```python
from build123d import *

# Parameters (mm, degrees)
EXTRUDE_2_DEPTH     = 9.8
CUT_EXTRUDE_1_DEPTH = 3
CUT_EXTRUDE_2_DEPTH = 2.5


with BuildPart() as part:
    # 草图1 → 凸台-拉伸2 (new body)
    with BuildSketch(Plane(origin=(0, 0, 0), x_dir=(1, 0, 0), z_dir=(0, 1, 0))):
        with BuildLine():
            Line((4.583240997, 11.690443213), (4.583240997, 14.234072022))
            Line((4.583240997, 14.234072022), (1.518891733, 14.234072022))
            ThreePointArc((1.518891733, 14.234072022), (-1.351843031, 11.65188196), (-2.416759003, 7.940443213))
            Line((-2.416759003, 7.940443213), (-2.416759003, 5.734072022))
            Line((-2.416759003, 5.734072022), (-5.066759003, 5.734072022))
            Line((-5.066759003, 5.734072022), (-5.066759003, -14.065927978))
            Line((-5.066759003, -14.065927978), (-3.166759003, -14.065927978))
            Line((-3.166759003, -14.065927978), (-3.166759003, -7.864819945))
            ThreePointArc((-3.166759003, -7.864819945), (-0.896836557, -2.38474239), (4.583240997, -0.114819945))
            Line((4.583240997, -0.114819945), (4.583240997, 4.190443213))
            ThreePointArc((4.583240997, 4.190443213), (0.833240997, 7.940443213), (4.583240997, 11.690443213))
        make_face()
        with BuildLine():
            ThreePointArc((11.583240997, 7.940443213), (10.518325026, 11.65188196), (7.647590262, 14.234072022))
            Line((7.647590262, 14.234072022), (4.583240997, 14.234072022))
            Line((4.583240997, 14.234072022), (4.583240997, 11.690443213))
            ThreePointArc((4.583240997, 11.690443213), (7.234891427, 10.592093643), (8.333240997, 7.940443213))
            ThreePointArc((8.333240997, 7.940443213), (7.234891427, 5.288792784), (4.583240997, 4.190443213))
            Line((4.583240997, 4.190443213), (4.583240997, -0.114819945))
            ThreePointArc((4.583240997, -0.114819945), (10.063318551, -2.38474239), (12.333240997, -7.864819945))
            Line((12.333240997, -7.864819945), (12.333240997, -14.065927978))
            Line((12.333240997, -14.065927978), (14.233240997, -14.065927978))
            Line((14.233240997, -14.065927978), (14.233240997, 5.734072022))
            Line((14.233240997, 5.734072022), (11.583240997, 5.734072022))
            Line((11.583240997, 5.734072022), (11.583240997, 7.940443213))
        make_face()
    extrude(amount=EXTRUDE_2_DEPTH)

    # 草图2 → 切除-拉伸1 (cut)
    with BuildSketch(Plane(origin=(0, 9.8, 0), x_dir=(1, 0, 0), z_dir=(0, 1, 0))):
        Polygon((-7.578838201, -4.016286107), (16.085093039, -4.259527691), (16.085093039, 14.991306239), (-7.578838201, 14.991306239), align=None)
    extrude(amount=-CUT_EXTRUDE_1_DEPTH, mode=Mode.SUBTRACT)

    # 草图3 → 切除-拉伸2 (cut)
    with BuildSketch(Plane(origin=(0, 6.8, 0), x_dir=(1, 0, 0), z_dir=(0, 1, 0))):
        Polygon((-9.750638057, 0), (19.90166932, 0), (19.90166932, 15.470839647), (-9.750638057, 15.762729548), align=None)
    extrude(amount=-CUT_EXTRUDE_2_DEPTH, mode=Mode.SUBTRACT)


solid = part.part
```
Work out the finished part from the listing and answer in its coordinate system (mm). A direction names the side the tool comes from. Round coordinates to 2 decimals unless told otherwise and drop trailing zeros. Write each loop counter-clockwise with the first axis right and the second up, starting at its lowest first coordinate (ties: lowest second). Pieces come first, ordered by that corner, then holes. Notation, with made-up numbers: (-5.75, -37) - (22.25, -37) arc R30 ccw to (22.25, -2) - close; hole circle Ø5 at (41.25, -36.75). An arc over 180 degrees is marked (long way). Return JSON: item names as keys, results as strings. Group by question number.
Q1. The part is cut by section D-D on x = 5.75. Write down the section's boundary in (y, z), then the cut area to 3 significant figures.
Q2. The part is cut by section C-C on y = 8.25. Write down the section's boundary in (x, z).
Q3. The part is cut by section A-A on y = 1.5. Write down the section's boundary in (x, z), then the cut area to 3 significant figures.
Q4. The part is cut by section B-B on z = 9.75. Write down the section's boundary in (x, y).
Q5. For faces 1 (the flat face through (13, 2, -5.734)), 2 (the flat face through (-4, 5, 14.066)), 3 (the flat face through (4, 4.3, -4)), 4 (the flat face through (-3.167, 5, 11)), 5 (the flat face through (-2.417, 2, -7)), determine the directions among +Z, -Z, +X, -X, +Y, -Y from which every point of the face is accessible in a straight line to the end or side of a thin tool.
Q6. Each of these flat-tipped pins is pushed along its axis until it touches: pin 1 Ø4 at (y, z) = (1.5, -8) entering from +X; pin 2 Ø5 at (x, y) = (3.5, 7.5) entering from -Z; pin 3 Ø2 at (x, y) = (-4.5, 2) entering from -Z; pin 4 Ø3.5 at (x, z) = (3, 3) entering from +Y. Where does it stop, or does it pass through?
Q7. Find the intervals of material crossed by L1, parallel to Z at x = 4.5, y = 2.75; L2, parallel to X at y = 8.25, z = 8.5; L3, parallel to Z at x = -3.75, y = 1.5, in increasing order.
Solved:
{
 "1": {"outline": "(0, -14.23) - (4.3, -14.23) - (4.3, -11.5) - (0, -11.5) - close; (0, -4.38) - (4.3, -4.38) - (4.3, 0) - (6.8, 0) - (6.8, 0.2) - (0, 0.2) - close", "area": "31.9 mm²"},
 "2": {"outline": "(-5.07, 4.04) - (-2.18, 4.07) arc R7.75 cw to (-3.17, 7.86) - (-3.17, 14.07) - (-5.07, 14.07) - close; (11.42, 4.21) - (14.23, 4.24) - (14.23, 14.07) - (12.33, 14.07) - (12.33, 7.86) arc R7.75 cw to start"},
 "3": {"outline": "(-5.07, -5.73) - (-2.42, -5.73) - (-2.42, -7.94) arc R7 ccw to (1.52, -14.23) - (7.65, -14.23) arc R7 ccw to (11.58, -7.94) - (11.58, -5.73) - (14.23, -5.73) - (14.23, 14.07) - (12.33, 14.07) - (12.33, 7.86) arc R7.75 cw to (-3.17, 7.86) - (-3.17, 14.07) - (-5.07, 14.07) - close; hole circle Ø7.5 at (4.58, -7.94)", "area": "252 mm²"},
 "4": {"outline": "(-5.07, 0) - (-3.17, 0) - (-3.17, 9.8) - (-5.07, 9.8) - close; (12.33, 0) - (14.23, 0) - (14.23, 9.8) - (12.33, 9.8) - close"},
 "5": {"face 1": "-Z, +X, +Y, -Y", "face 2": "+Z, +X, -X, +Y, -Y", "face 3": "-Z, +X, -X, +Y", "face 4": "+Z, +Y, -Y", "face 5": "-Z, -X, +Y, -Y"},
 "6": {"pin 1": "x = 11.58", "pin 2": "z = 0", "pin 3": "z = -5.73", "pin 4": "through"},
 "7": {"L1": "-14.23 to -11.69, -4.19 to 0.12", "L2": "-5.07 to -3.17, 12.33 to 14.23", "L3": "-5.73 to 14.07"}
}
